Source: CAD feature listing. Evaluate the final solid. Frame: model axes, mm. A direction names the side the tool comes from. Round coordinates to 2 decimals unless told otherwise and drop trailing zeros. Loops run counter-clockwise (first coordinate to the right, second up) from the corner with the lowest first, then second, coordinate; pieces in that order, holes last.
(1) Section A-A, the plane y = 34.5. Return the cut outline in (x, z).
(2) Set-up query: faces 1 (the cylindrical face through (15.47, 92.71, 20.39)), 2 (the flat face through (42.3, 19.2, -5.5)), 3 (the flat face through (-5, 0, 0)). Return all of +Z, -Z, +X, -X, +Y, -Y with unobstructed straight access to the full face (end or side cutting, diameter ignored); none if empty.
(3) Section B-B, the plane z = 14. Return the cut outline in (x, y), plus the area to 3 significant figures.
(4) First-contact query: pin 1 Ø5 at (x, z) = (-7, -16) entering from +Y; pin 2 Ø5 at (y, z) = (80, 8.5) entering from +X; pin 3 Ø1 at (y, z) = (-2.5, -9.5) entering from +X; pin 4 Ø1.8 at (x, z) = (-38.62, -21) entering from -Y. Flat tips, straight axial feed; report the tip coordinate or a pass-through.
(5) Material intervals for probe 1 along X at (y, z) = (-1.4, -21); probe 2 along Y at (x, z) = (-5.5, -17.5); probe 3 along Y at (x, z) = (2, -1.5), sorted ascending.
(6) Mould query, pull axis Z, two halves, no side actions, for faces 4 (the flat face through (35, 36, 25)), 5 (the cylindrical face through (15.47, 92.71, -20.39)), 6 (the cylindrical face through (44.06, 2.69, 0.05)), 7 (the flat face through (42.3, 19.1, 3.5)). Classes: pulls with the +Z half, pulls with the -Z half, needs draft (parallel to the pull), parting line crosses it, or undercut.
(7) Section C-C, the plane z = -0.5. Return the cut outline in (x, y), plus the area to 3 significant figures.
```python
from build123d import *

# Parameters (mm, degrees)
EXTRUDE_1_DEPTH       = 25
SKETCH_4_R            = 22
CUT_EXTRUDE_1_DEPTH   = 1.8
CUT_EXTRUDE_START     = 5.5
CUT_EXTRUDE_1_2_DEPTH = 2
CUT_EXTRUDE_2_REACH   = 124.068
SKETCH_5_R            = 1
CUT_EXTRUDE_3_REACH   = 112.991
SKETCH_6_R            = 1
CUT_EXTRUDE_1_3_DEPTH = 1.8
SKETCH_8_W            = 1.7
SKETCH_8_H            = 9.2
EXTRUDE_1_2_DEPTH     = 1.7
CUT_EXTRUDE_2_2_DEPTH = 2
SKETCH_14_W           = 13.81884782
SKETCH_14_H           = 18.9
CUT_EXTRUDE_3_2_DEPTH = 1.8
EXTRUDE_2_DEPTH       = 1.8
SKETCH_16_W           = 4
SKETCH_16_H           = 2.04
CUT_EXTRUDE_4_DEPTH   = 1.2


with BuildPart() as part:
    # 草图2 → Extrude 1 (new, symmetric)
    with BuildSketch(Plane.XY):
        with BuildLine():
            Line((-42.61884782, 0), (33.310872136, 0))
            ThreePointArc((33.310872136, 0), (41.502392579, 4.264235636), (42.707798344, 13.420201433))
            Line((42.707798344, 13.420201433), (12.398479455, 96.694370679))
            Line((12.398479455, 96.694370679), (15.217557318, 97.720431109))
            Line((15.217557318, 97.720431109), (45.526876206, 14.446261863))
            ThreePointArc((45.526876206, 14.446261863), (43.959848712, 2.543506327), (33.310872136, -3))
            Line((33.310872136, -3), (-42.61884782, -3))
            Line((-42.61884782, -3), (-42.61884782, 0))
        make_face()
    extrude(amount=EXTRUDE_1_DEPTH, both=True)

    # 草图4 → Cut-Extrude 1 (cut)
    with BuildSketch(Plane(origin=(44.844182434, 16.321947586, 0), x_dir=(0, 0, -1), z_dir=(0.939692620785907, 0.3420201433256728, 0))):
        with Locations(Location((0, 61.222456878, 0), (0, 0, 90))):
            Circle(SKETCH_4_R)
    extrude(amount=-CUT_EXTRUDE_1_DEPTH, mode=Mode.SUBTRACT)

    # 草图3 → Cut-Extrude 1 2 (cut)
    with BuildSketch(Plane.XY.offset(CUT_EXTRUDE_START)):
        with BuildLine():
            Line((8.762964592, -1.2), (33.310872136, -1.2))
            ThreePointArc((33.310872136, -1.2), (42.485375032, 3.575943913), (43.835429489, 13.830625605))
            Line((43.835429489, 13.830625605), (29.737865394, 52.563364626))
            Line((29.737865394, 52.563364626), (28.711804964, 55.382442488))
            Line((28.711804964, 55.382442488), (30.403251681, 55.998078746))
            Line((30.403251681, 55.998078746), (31.429312111, 53.179000884))
            Line((31.429312111, 53.179000884), (45.526876206, 14.446261863))
            ThreePointArc((45.526876206, 14.446261863), (43.959848712, 2.543506327), (33.310872136, -3))
            Line((33.310872136, -3), (8.762964592, -3))
            Line((8.762964592, -3), (8.762964592, -1.2))
        make_face()
    cut_extrude_1_2 = extrude(amount=-CUT_EXTRUDE_1_2_DEPTH, mode=Mode.SUBTRACT)

    # 镜向1: Cut-Extrude 1 2 across plane
    add(cut_extrude_1_2.mirror(Plane.XY), mode=Mode.SUBTRACT)

    # 草图5 → Cut-Extrude 2 (cut, up to next)
    with BuildSketch(Plane(origin=(44.844182434, 16.321947586, 0), x_dir=(0, 0, -1), z_dir=(0.939692620785907, 0.3420201433256728, 0)), mode=Mode.PRIVATE) as cut_extrude_2_sk1:
        with Locations(Location((-21, 82.622456878, 0), (0, 0, 90))):
            Circle(SKETCH_5_R)
    cut_extrude_2_tool1 = extrude(cut_extrude_2_sk1.sketch, amount=-CUT_EXTRUDE_2_REACH, mode=Mode.PRIVATE) & part.part
    cut_extrude_2 = cut_extrude_2_tool1.solids().sort_by_distance((16.585638, 93.961661, 21))[0]
    add(cut_extrude_2, mode=Mode.SUBTRACT)

    # 镜向2: Cut-Extrude 2 across plane
    add(cut_extrude_2.mirror(Plane.XY), mode=Mode.SUBTRACT)

    # 草图6 → Cut-Extrude 3 (cut, up to next)
    with BuildSketch(Plane(origin=(0, 0, 0), x_dir=(1, 0, 0), z_dir=(0, 1, 0)), mode=Mode.PRIVATE) as cut_extrude_3_sk1:
        with Locations(Location((-38.61884782, -21, 0), (0, 0, 270))):
            Circle(SKETCH_6_R)
    cut_extrude_3_tool1 = extrude(cut_extrude_3_sk1.sketch, amount=-CUT_EXTRUDE_3_REACH, mode=Mode.PRIVATE) & part.part
    cut_extrude_3 = cut_extrude_3_tool1.solids().sort_by_distance((-38.618848, 0, 21))[0]
    add(cut_extrude_3, mode=Mode.SUBTRACT)

    # 镜向3: Cut-Extrude 3 across plane
    add(cut_extrude_3.mirror(Plane.XY), mode=Mode.SUBTRACT)

    # 草图7 → Cut-Extrude 1 3 (cut)
    with BuildSketch(Plane.XZ.offset(3)):
        Polygon((-40.91884782, -5.9), (-26.91884782, -5.9), (-26.91884782, 5.9), (-40.91884782, 5.9), (-40.91884782, 4.6), (-42.61884782, 4.6), (-42.61884782, -4.6), (-40.91884782, -4.6), align=None)
    extrude(amount=-CUT_EXTRUDE_1_3_DEPTH, mode=Mode.SUBTRACT)

    # 草图8 → Extrude 1 2 (add)
    with BuildSketch(Plane.XZ.offset(1.2)):
        with Locations((-41.76884782, 0)):
            Rectangle(SKETCH_8_W, SKETCH_8_H)
    extrude(amount=EXTRUDE_1_2_DEPTH)

    # 草图12 → Cut-Extrude 2 2 (cut)
    with BuildSketch(Plane.XZ.offset(3)):
        Polygon((-10.1, -8.1), (-10.1, -10.6), (15.1, -10.6), (15.1, 10.6), (-10.1, 10.6), (-10.1, 8.1), (-13.1, 8.1), (-13.1, -8.1), align=None)
    extrude(amount=-CUT_EXTRUDE_2_2_DEPTH, mode=Mode.SUBTRACT)

    # 草图14 → Cut-Extrude 3 2 (cut)
    with BuildSketch(Plane.XZ.offset(3)):
        with Locations((-20.00942391, 1.35)):
            Rectangle(SKETCH_14_W, SKETCH_14_H)
    extrude(amount=-CUT_EXTRUDE_3_2_DEPTH, mode=Mode.SUBTRACT)

    # 草图15 → 凸台-拉伸2 (add)
    with BuildSketch(Plane.XZ.offset(1.2)):
        Polygon((-25.30942391, 6.1), (-14.60942391, 6.1), (-14.60942391, 10.8), (-15.60942391, 10.8), (-15.60942391, 7.1), (-24.30942391, 7.1), (-24.30942391, 10.8), (-25.30942391, 10.8), align=None)
    extrude(amount=EXTRUDE_2_DEPTH)

    # 草图16 → 切除-拉伸4 (cut)
    with BuildSketch(Plane(origin=(0, 0, 0), x_dir=(1, 0, 0), z_dir=(0, 1, 0))):
        with Locations((-19.95942391, -8.95)):
            Rectangle(SKETCH_16_W, SKETCH_16_H)
    extrude(amount=-CUT_EXTRUDE_4_DEPTH, mode=Mode.SUBTRACT)


solid = part.part
```
Output values:
1. outline: (35.04, -25) - (38.23, -25) - (38.23, -5.5) - (36.31, -5.5) - (36.31, -3.5) - (38.23, -3.5) - (38.23, 3.5) - (36.31, 3.5) - (36.31, 5.5) - (38.23, 5.5) - (38.23, 25) - (35.04, 25) - close
2. face 1: none
2. face 2: +X
2. face 3: +Z, -Z, -X
3. outline: (-42.62, -3) - (33.31, -3) arc R13 ccw to (45.53, 14.45) - (29.71, 57.91) - (28.02, 57.29) - (16.41, 89.18) - (18.1, 89.8) - (15.22, 97.72) - (12.4, 96.69) - (42.71, 13.42) arc R10 cw to (33.31, 0) - (-42.62, 0) - close
3. area: 499 mm2
4. pin 1: stops at y = 0
4. pin 2: stops at x = 20.66
4. pin 3: stops at x = 38.31
4. pin 4: passes through
5. probe 1: x = -42.62 to -39.62, -37.62 to 39.56
5. probe 2: y = -3 to 0
5. probe 3: y = -1 to 0
6. face 4: pulls with the +Z half
6. face 5: undercut
6. face 6: needs draft
6. face 7: undercut
7. outline: (-42.62, -2.9) - (-40.92, -2.9) - (-40.92, -1.2) - (-13.1, -1.2) - (-13.1, -1) - (15.1, -1) - (15.1, -3) - (33.31, -3) arc R13 ccw to (45.53, 14.45) - (31.43, 53.18) - (29.74, 52.57) - (14.69, 93.9) - (16.38, 94.52) - (15.22, 97.72) - (12.4, 96.69) - (42.71, 13.42) arc R10 cw to (33.31, 0) - (-42.62, 0) - close
7. area: 374 mm2
